from build123d import *

# Parameters (mm, degrees)
BOSS_EXTRUDE1_DEPTH = 19
FILLET1_R           = 3
FILLET2_R           = 10
FILLET3_R           = 3


with BuildPart() as part:
    # Sketch1 → Boss-Extrude1 (new, symmetric)
    with BuildSketch(Plane(origin=(0, 0, 0), x_dir=(1, 0, 0), z_dir=(0, 1, 0))):
        Polygon((0, 0), (0, -19), (79, -19), (79, -20), (-1, -20), (-1, 0), align=None)
    extrude(amount=BOSS_EXTRUDE1_DEPTH, both=True)

    # Fillet1
    fillet1_edges = [part.edges().sort_by_distance(p)[0] for p in [
        (79, 19, 19.5),
        (79, -19, 19.5),
    ]]
    fillet(fillet1_edges, radius=FILLET1_R)

    # Fillet2
    fillet2_edges = [part.edges().sort_by_distance(p)[0] for p in [
        (0, 0, 19),
        (-1, 0, 20),
    ]]
    fillet(fillet2_edges, radius=FILLET2_R)

    # Sketch2 → Revolve2 (revolve)
    with BuildSketch(Plane(origin=(0, 0, 0), x_dir=(1, 0, 0), z_dir=(0, 1, 0))):
        with BuildLine():
            Line((-0.773743612, -3), (-15.773743612, -3))
            ThreePointArc((-15.773743612, -3), (-24.25464239, 2.469780889), (-30.503131217, -5.454897934))
            Line((-30.503131217, -5.454897934), (-0.503131217, -5.454897934))
            Line((-0.503131217, -5.454897934), (-0.773743612, -3))
        make_face()
    revolve(axis=Axis((-0.503131217, 0, 5.454897934), (-1, 0, 0)))

    # Fillet3
    fillet3_edges = [part.edges().sort_by_distance(p)[0] for p in [
        (-15.773743612, 0, 7.909795868),
        (-1, 0, 7.909795868),
    ]]
    fillet(fillet3_edges, radius=FILLET3_R - 0.0001)  # a hair under: the kernel refuses the full size


solid = part.part
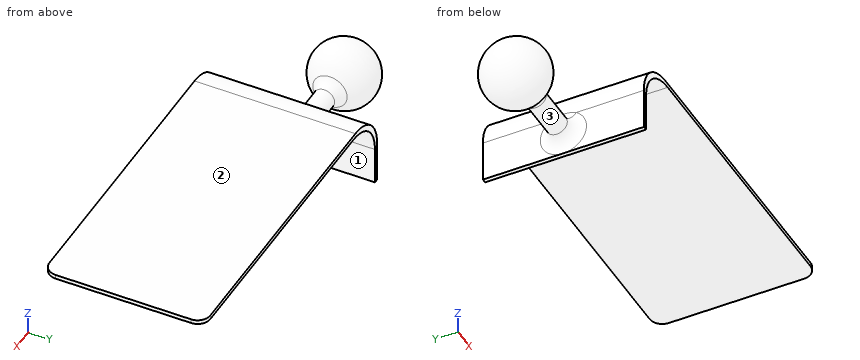
Check sheet for the modelled part. Datum: model origin and axes. Units: mm. Face numbers are marked on the shaded views. A direction names the side the tool comes from. Coordinates: 2 decimals unless noted, no trailing zeros. Write each loop counter-clockwise with the first axis right and the second up, starting at its lowest first coordinate (ties: lowest second). Pieces come first, ordered by that corner, then holes. Notation, with made-up numbers: M 60.25,44 L 114.25,44 A21 cw 114.25,59 Z; hole C 50,82 d7. An arc over 180 degrees is marked long. Answer as CSV lines item,"result".
Q1. Cross-section at A-A (y = 15). Record the boundary of the cut face in (x, z), then the cut area to 3 significant figures.
Check result:
outline,"M -1,0 L 0,0 L 0,9 A10 cw 10,19 L 79,19 L 79,20 L 9,20 A10 ccw -1,10 Z"
area,"99.0 mm^2"
Q2. Material ranges on probe 1 along X at (y, z) = (7.5, 1.75); probe 2 along Z at (x, y) = (36, 17.5); probe 3 along X at (y, z) = (1, 8.5), recorded low to high. Write a range as from..to.
Check result:
probe 1,"-1..0"
probe 2,"19..20"
probe 3,"-30.03..-15.73, -2..0"
Q3. Cross-section at C-C (z = 18). Record the boundary of the cut face in (x, y).
Check result:
outline,"M 3,-19 L 5.64,-19 L 5.64,19 L 3,19 Z"
Q4. Cross-section at D-D (x = 23). Record the boundary of the cut face in (y, z), then the cut area to 3 significant figures.
Check result:
outline,"M -19,19 L 19,19 L 19,20 L -19,20 Z"
area,"38.0 mm^2"
Q5. Cross-section at B-B (x = -7). Record the boundary of the cut face in (y, z).
Check result:
outline,"C 0,5.45 d4.91"
Q6. Set-up check for the marked faces 1, 2 and 3: record each of +Z, -Z, +X, -X, +Y, -Y from which the full face is reachable in a straight line by a thin tool's end or side.
Check result:
face 1,"-Z, +X, +Y, -Y"
face 2,"+Z, +X, -X, +Y, -Y"
face 3,"none"
Q7. Go/stop test with flat-tipped pins: pin 1 (4 mm diameter, centred on x = -12.5, z = 5.5, fed in from +Y); pin 2 (1.1 mm diameter, centred on x = -0.5, y = -1, fed in from -Z); pin 3 (5 mm diameter, centred on y = 1, z = 1.5, fed in from -X). Record where each tip stops, or that it passes through.
Check result:
pin 1,"y = 2.55"
pin 2,"z = 0"
pin 3,"x = -30.45"
